from build123d import *

# Parameters (mm, degrees)
SKETCH1_W           = 110
SKETCH1_H           = 80
SKETCH1_R           = 2.75
SKETCH1_R_2         = 1.25
SKETCH1_R_3         = 2.1
BOSS_EXTRUDE1_DEPTH = 5
SKETCH2_R           = 2.1
CUT_EXTRUDE1_DEPTH  = 69.190908485
SKETCH7_W           = 20
SKETCH7_H           = 40
BOSS_EXTRUDE2_DEPTH = 5
CUT_EXTRUDE2_REACH  = 99.211
SKETCH8_R           = 1.75


with BuildPart() as part:
    # Sketch1 → Boss-Extrude1 (new body)
    with BuildSketch(Plane(origin=(0, 0, 0), x_dir=(1, 0, 0), z_dir=(0, 1, 0))):
        Rectangle(SKETCH1_W, SKETCH1_H)
        with Locations(Location((-18, 16, 0), (0, 0, 270))):
            Circle(SKETCH1_R, mode=Mode.SUBTRACT)
        with Locations(Location((18, 16, 0), (0, 0, 270))):
            Circle(SKETCH1_R, mode=Mode.SUBTRACT)
        with Locations(Location((18, -16, 0), (0, 0, 270))):
            Circle(SKETCH1_R, mode=Mode.SUBTRACT)
        with Locations(Location((-18, -16, 0), (0, 0, 270))):
            Circle(SKETCH1_R, mode=Mode.SUBTRACT)
        with Locations(Location((-22, 26, 0), (0, 0, 270))):
            Circle(SKETCH1_R_2, mode=Mode.SUBTRACT)
        with Locations(Location((22, 26, 0), (0, 0, 270))):
            Circle(SKETCH1_R_2, mode=Mode.SUBTRACT)
        with Locations(Location((-24, -26, 0), (0, 0, 270))):
            Circle(SKETCH1_R_3, mode=Mode.SUBTRACT)
        with Locations(Location((24, -26, 0), (0, 0, 270))):
            Circle(SKETCH1_R_3, mode=Mode.SUBTRACT)
    extrude(amount=BOSS_EXTRUDE1_DEPTH)

    # Sketch2 → Cut-Extrude1 (cut, through all)
    with BuildSketch(Plane(origin=(0, 5, 0), x_dir=(1, 0, 0), z_dir=(0, 1, 0))):
        with Locations(Location((-46, 10, 0), (0, 0, 270))):
            Circle(SKETCH2_R)
        with Locations(Location((-46, -10, 0), (0, 0, 270))):
            Circle(SKETCH2_R)
        with Locations(Location((46, -10, 0), (0, 0, 270))):
            Circle(SKETCH2_R)
        with Locations(Location((46, 10, 0), (0, 0, 270))):
            Circle(SKETCH2_R)
        with BuildLine():
            Line((-38, 4), (-38, -4))
            ThreePointArc((-38, -4), (-40, -6), (-42, -4))
            Line((-42, -4), (-42, 4))
            ThreePointArc((-42, 4), (-40, 6), (-38, 4))
        make_face()
        with BuildLine():
            Line((42, 4), (42, -4))
            ThreePointArc((42, -4), (40, -6), (38, -4))
            Line((38, -4), (38, 4))
            ThreePointArc((38, 4), (40, 6), (42, 4))
        make_face()
    extrude(amount=-CUT_EXTRUDE1_DEPTH, mode=Mode.SUBTRACT)

    # Sketch7 → Boss-Extrude2 (add)
    with BuildSketch(Plane(origin=(0, 0, 0), x_dir=(1, 0, 0), z_dir=(0, 1, 0))):
        with Locations((-45, 60)):
            Rectangle(SKETCH7_W, SKETCH7_H)
    extrude(amount=BOSS_EXTRUDE2_DEPTH)

    # Sketch8 → Cut-Extrude2 (cut, up to next)
    with BuildSketch(Plane(origin=(0, 5, 0), x_dir=(1, 0, 0), z_dir=(0, 1, 0)), mode=Mode.PRIVATE) as cut_extrude2_sk1:
        with Locations(Location((-51, 75, 0), (0, 0, 270))):
            Circle(SKETCH8_R)
    cut_extrude2_tool1 = extrude(cut_extrude2_sk1.sketch, amount=-CUT_EXTRUDE2_REACH, mode=Mode.PRIVATE) & part.part
    # Sketch8 → Cut-Extrude2 (cut, up to next)
    with BuildSketch(Plane(origin=(0, 5, 0), x_dir=(1, 0, 0), z_dir=(0, 1, 0)), mode=Mode.PRIVATE) as cut_extrude2_sk2:
        with Locations(Location((-43, 75, 0), (0, 0, 270))):
            Circle(SKETCH8_R)
    cut_extrude2_tool2 = extrude(cut_extrude2_sk2.sketch, amount=-CUT_EXTRUDE2_REACH, mode=Mode.PRIVATE) & part.part
    add(cut_extrude2_tool1.solids().sort_by_distance((-51, 5, -75))[0], mode=Mode.SUBTRACT)
    add(cut_extrude2_tool2.solids().sort_by_distance((-43, 5, -75))[0], mode=Mode.SUBTRACT)


solid = part.part
Build history of the part. All positions in model axes, mm. A direction names the side the tool comes from. Round coordinates to 2 decimals unless told otherwise and drop trailing zeros. Write each loop counter-clockwise with the first axis right and the second up, starting at its lowest first coordinate (ties: lowest second). Pieces come first, ordered by that corner, then holes. Notation, with made-up numbers: M 52.25,24.25 L 69.25,24.25 A30 cw 69.25,60.25 Z; hole C -15.75,41.25 d5. An arc over 180 degrees is marked long. Use CSV: the item, a comma, the result in double quotes.
1. Wall check: probe 1 along X at (y, z) = (2.9, -26); probe 2 along X at (y, z) = (3.6, 16); probe 3 along X at (y, z) = (3.85, -52). Give the ranges that are in metal, low to high. Write a range as from..to.
Reply:
probe 1,"x = -55..-23.25, -20.75..20.75, 23.25..55"
probe 2,"x = -55..-20.75, -15.25..15.25, 20.75..55"
probe 3,"x = -55..-35"
2. Two-plate mould, pull along Z, no slides. Class faces 1 (the face through (40, 3, -6)), 2 (the face through (-55, 2, -19)), 3 (the face through (-1, 2, 40)): +Z half, -Z half, draft (parallel to the pull), parting line (faces both ways), or undercut.
Reply:
face 1,"undercut"
face 2,"draft"
face 3,"+Z half"
3. Saw through at D-D (y = 2.3). State how many separate pieces and enclosed holes the cut face has, plus the area to 3 significant figures.
Reply:
separate pieces,"1"
enclosed holes,"16"
area,"9,300 mm²"
4. Tool access for faces 4 (the face through (-35, 2, -60)), 5 (the face through (55, 2, 1)), 6 (the face through (38, 3, 0)): list every direction of +Z, -Z, +X, -X, +Y, -Y with a clear straight run to the whole face (end or side of a thin tool).
Reply:
face 4,"-Z, +X, +Y, -Y"
face 5,"+Z, -Z, +X, +Y, -Y"
face 6,"+Y, -Y"
5. Saw through at C-C (x = -51). Give the cut face in (y, z).
Reply:
outline,"M 0,-80 L 5,-80 L 5,-76.75 L 0,-76.75 Z; M 0,-73.25 L 5,-73.25 L 5,40 L 0,40 Z"
6. Saw through at B-B (z = 15). Give the cut face in (x, y).
Reply:
outline,"M -55,0 L -20.56,0 L -20.56,5 L -55,5 Z; M -15.44,0 L 15.44,0 L 15.44,5 L -15.44,5 Z; M 20.56,0 L 55,0 L 55,5 L 20.56,5 Z"
7. Flat gauge pins, fed straight in: pin 1 (2.5 mm diameter, centred on x = -46, z = -10, fed in from +Y); pin 2 (1.5 mm diameter, centred on y = 2.5, z = -55, fed in from +X); pin 3 (2 mm diameter, centred on x = 34.5, y = 3.5, fed in from -Z). Where does each tip first touch, or does it go through?
Reply:
pin 1,"passes through"
pin 2,"stops at x = -35"
pin 3,"stops at z = -40"
8. Saw through at A-A (x = -18). Give the cut face in (y, z).
Reply:
outline,"M 0,-40 L 5,-40 L 5,-18.75 L 0,-18.75 Z; M 0,-13.25 L 5,-13.25 L 5,13.25 L 0,13.25 Z; M 0,18.75 L 5,18.75 L 5,40 L 0,40 Z"
